Design review of the part built by this model. Coordinates are the model's own, in mm. A direction names the side the tool comes from. Give positions to 0.01 mm unless a question says otherwise; leave off trailing zeros. Write each loop counter-clockwise with the first axis right and the second up, starting at its lowest first coordinate (ties: lowest second). Pieces come first, ordered by that corner, then holes. Notation, with made-up numbers: M 6.25,62.25 L 37.25,62.25 A16 ccw 37.25,88.25 Z; hole C 25,84 d6. An arc over 180 degrees is marked long. Answer in a Markdown table with one row per item.
```python
from build123d import *

# Parameters (mm, degrees)
PAD001_DEPTH                  = 3
SKETCH002_W                   = 5
SKETCH002_H                   = 3
PAD002_DEPTH                  = 3
SKETCH006_W                   = 1.5
SKETCH006_H                   = 4
POCKET002_DEPTH               = 169.48223
SKETCH006_MIRRORED004_2_W     = 1.5
SKETCH006_MIRRORED004_2_H     = 4
POCKET002_MIRRORED004_2_DEPTH = 169.48223
SKETCH008_R                   = 1.9
POCKET003_DEPTH               = 3.001
SKETCH013_R                   = 1.9
POCKET007_DEPTH               = 169.48223
SKETCH038_R                   = 1.9
POCKET025_DEPTH               = 169.48223


with BuildPart() as part:
    # Sketch001 → Pad001 (new body)
    with BuildSketch(Plane.XY):
        with BuildLine():
            Line((-19, 32.25), (-19, -32.25))
            Line((-19, -32.25), (-9.375, -32.25))
            Line((-9.375, -32.25), (-9.375, 27.75))
            Line((-9.375, 27.75), (9.375, 27.75))
            Line((9.375, 27.75), (9.375, -32.25))
            Line((9.375, -32.25), (19, -32.25))
            Line((19, -32.25), (19, 32.25))
            ThreePointArc((19, 32.25), (17.096194, 36.846194), (12.5, 38.75))
            Line((-12.5, 38.75), (12.5, 38.75))
            ThreePointArc((-12.5, 38.75), (-17.096194, 36.846194), (-19, 32.25))
        make_face()
    extrude(amount=PAD001_DEPTH)

    # Sketch002 (on DatumPlane) → Pad002 (join)
    with BuildSketch(Plane.XZ.offset(32.25)):
        with Locations((-11.875, 1.5)):
            Rectangle(SKETCH002_W, SKETCH002_H)
        with Locations((11.875, 1.5)):
            Rectangle(SKETCH002_W, SKETCH002_H)
    extrude(amount=PAD002_DEPTH)

    # Sketch006 (on Face14 of Pad002) → Pocket002 (cut, through all)
    with BuildSketch(Plane.XY.offset(3)):
        with Locations((-13.125, 16.75)):
            Rectangle(SKETCH006_W, SKETCH006_H)
    pocket002 = extrude(amount=-POCKET002_DEPTH, mode=Mode.SUBTRACT)

    # Sketch006 Mirrored004 2 → Pocket002 Mirrored004 2 (cut, through all)
    with BuildSketch(Plane(origin=(0, 0, 3), x_dir=(-1, 0, 0), z_dir=(0, 0, -1))):
        with Locations((-13.125, 16.75)):
            Rectangle(SKETCH006_MIRRORED004_2_W, SKETCH006_MIRRORED004_2_H)
    pocket002_mirrored004_2 = extrude(amount=POCKET002_MIRRORED004_2_DEPTH, mode=Mode.SUBTRACT)

    # Mirrored005: Pocket002, Pocket002 Mirrored004 2 across Sketch006 H_Axis
    add(pocket002.mirror(Plane(origin=(0, 0, 3), x_dir=(0, 0, 1), z_dir=(0, 1, 0))), mode=Mode.SUBTRACT)
    add(pocket002_mirrored004_2.mirror(Plane(origin=(0, 0, 3), x_dir=(0, 0, 1), z_dir=(0, 1, 0))), mode=Mode.SUBTRACT)

    # Sketch008 (on Face4 of MultiTransform002) → Pocket003 (cut, through all)
    with BuildSketch(Plane.XY.offset(3)):
        with Locations((-7.25, 32.75)):
            Circle(SKETCH008_R)
        with Locations((7.25, 32.75)):
            Circle(SKETCH008_R)
    extrude(amount=-POCKET003_DEPTH, mode=Mode.SUBTRACT)

    # Sketch013 (on Face4 of Pocket003) → Pocket007 (cut, through all)
    with BuildSketch(Plane.XY.offset(3)):
        with Locations((-14.1875, -5.25)):
            Circle(SKETCH013_R)
    pocket007 = extrude(amount=-POCKET007_DEPTH, mode=Mode.SUBTRACT)

    # Mirrored008: Pocket007 across Sketch013 V_Axis
    add(pocket007.mirror(Plane(origin=(0, 0, 3), x_dir=(0, 0, 1), z_dir=(1, 0, 0))), mode=Mode.SUBTRACT)

    # Sketch038 (on Face4 of Mirrored008) → Pocket025 (cut, through all)
    with BuildSketch(Plane.XY.offset(3)):
        with Locations((-14.1875, 4.75)):
            Circle(SKETCH038_R)
    pocket025 = extrude(amount=-POCKET025_DEPTH, mode=Mode.SUBTRACT)

    # Mirrored021: Pocket025 across Sketch038 V_Axis
    add(pocket025.mirror(Plane(origin=(0, 0, 3), x_dir=(0, 0, 1), z_dir=(1, 0, 0))), mode=Mode.SUBTRACT)


with BuildPart() as part_1:
    # Body001 placement: moved
    add(part.part.moved(Location((-67, -49, 0))))


solid = part_1.part
```
1) Add section B-B (y = -79). Write out the cut boundary in (x, z) (3 decimals), and give its area (4 significant figures).
Geometry says:
| item | result |
|---|---|
| outline | M -86,0 L -76.375,0 L -76.375,3 L -86,3 Z; M -57.625,0 L -48,0 L -48,3 L -57.625,3 Z |
| area | 57.75 mm^2 |
2) Add section C-C (x = -59.75). Write out the cut boundary in (y, z).
Geometry says:
| item | result |
|---|---|
| outline | M -21.25,0 L -18.15,0 L -18.15,3 L -21.25,3 Z; M -14.35,0 L -10.25,0 L -10.25,3 L -14.35,3 Z |
3) The part is to be moulded in two halves that separate along X. For faces 4 (the face through (-54, -63.75, 2)), 5 (the face through (-67, -10.25, 1)), 6 (the face through (-86, -49, 1)), say which applies: released by +X, released by -X, zero draft, split by the parting line, or undercut.
Geometry says:
| item | result |
|---|---|
| face 4 | undercut |
| face 5 | zero draft |
| face 6 | released by -X |
4) Insertion check: P1, Ø0.9, axis at y = -82.5, z = 1.5, coming from the -X side (3 decimals). The pin has a flat end and moves straight along its axis. Give the tip position at first contact, or say it passes through.
Geometry says:
| item | result |
|---|---|
| P1 | x = -81.375 |
5) Add section A-A (y = -44.25). Write out the cut boundary in (x, z) (1 decimal), and give its area (4 significant figures).
Geometry says:
| item | result |
|---|---|
| outline | M -86,0 L -83.1,0 L -83.1,3 L -86,3 Z; M -79.3,0 L -76.4,0 L -76.4,3 L -79.3,3 Z; M -57.6,0 L -54.7,0 L -54.7,3 L -57.6,3 Z; M -50.9,0 L -48,0 L -48,3 L -50.9,3 Z |
| area | 34.95 mm^2 |
6) For faces 1 (the face through (-57.625, -52, 1)), 2 (the face through (-80, -30.25, 2)), 3 (the face through (-55, -47, 0)), list the 3-axis set-ups (+Z, -Z, +X, -X, +Y, -Y) from which the entire face can be reached by the end or side of a thin tool; tool diameter is ignored.
Geometry says:
| item | result |
|---|---|
| face 1 | +Z, -Z, -Y |
| face 2 | +Z, -Z |
| face 3 | -Z, +X, -X, +Y, -Y |
7) Add section D-D (z = 2.05). Count the separate pieces of the cut face and the enclosed holes in it, and give its area (3 significant figures).
Geometry says:
| item | result |
|---|---|
| separate pieces | 1 |
| enclosed holes | 10 |
| area | 1,490 mm^2 |
8) To check wall thickness, follow probe 1 along X at (y, z) = (-67, 2.7) (3 decimals); probe 2 along Y at (x, z) = (-74, 0.2); probe 3 along X at (y, z) = (-71, 2.6) (3 decimals). State the ranges of each line that lie inside material, in increasing order. Write a range as [from, to].
Geometry says:
| item | result |
|---|---|
| probe 1 | [-86, -80.875], [-79.375, -76.375], [-57.625, -54.625], [-53.125, -48] |
| probe 2 | [-21.25, -18.13], [-14.37, -10.25] |
| probe 3 | [-86, -76.375], [-57.625, -48] |
